Could you check a few things on this model? Use its own coordinates, in mm. A direction names the side the tool comes from. Give positions to 0.01 mm unless a question says otherwise; leave off trailing zeros. Loops run counter-clockwise (first coordinate to the right, second up) from the corner with the lowest first, then second, coordinate; pieces in that order, holes last. Notation, with made-up numbers: M 40.5,-10.5 L 70.5,-10.5 A13 ccw 70.5,-6.5 Z; hole C -37.75,20 d10. An arc over 180 degrees is marked long. Use a Markdown table: item, result. Add a question column.
1) We'd pull the mould along X, two halves only. Please class faces 1 (the conical face through (42.2, -134, -9.49)), 2 (the flat face through (97.95, -168.89, -79.07)), 3 (the flat face through (85, -148, -74)): +X half, -X half, draft (parallel to the pull), parting line (faces both ways), or undercut.
2) Suppose I cut it at A-A on x = 0. List the corners of the cut face in (y, z) for me, and give its area (3 significant figures).
3) If I drill on line 1 along Z through (x, y) = (-28, -61); line 2 along Z through (x, y) = (-81.5, -109.5); line 3 along X through (y, z) = (111, -77), over which ranges is the centre line in solid material (lowest first)? Write a range as [from, to].
4) Which directions (+Z, -Z, +X, -X, +Y, -Y) give clear straight access to the entire face, cutting with the end or side of a thin tool? Please do faces 4 (the flat face through (106, 118, -19)), 5 (the flat face through (112.732, 120.258, -59.177)), 6 (the flat face through (-155, -33, -19)), 7 (the flat face through (-161, 37.5, -58)).
5) Suppose I cut it at C-C on x = -170.5. List the corners of the cut face in (y, z) for me, and give its area (3 significant figures).
6) Will these pins go through, and if not, where does the flat tip stop? pin 1 Ø12 at (x, y) = (-144.5, 32.5) entering from +Z; pin 2 Ø5 at (x, z) = (-40, -2) entering from +Y; pin 3 Ø15 at (x, y) = (47, -147) entering from +Z.
7) Suppose I cut it at B-B on z = -49. List the corners of the cut face in (x, y) for me.
```python
from build123d import *

# Parameters (mm, degrees)
SKETCH1_R                    = 150
BOSS_EXTRUDE1_DEPTH          = 75
CHAMFER1_SIZE                = 10
BOSS_EXTRUDE2_START          = -75
BOSS_EXTRUDE2_DEPTH          = 10
CHAMFER2_SIZE                = 10
BOSS_EXTRUDE3_DEPTH          = 10
CIRPATTERN2_COUNT            = 3
CIRPATTERN2_COPY_1_DEPTH     = 10
CIRPATTERN2_COPY_2_DEPTH     = 10
CHAMFER2_OF_CIRPATTERN2_SIZE = 10
SKETCH4_R                    = 110
BOSS_EXTRUDE4_DEPTH          = 9
BOSS_EXTRUDE4_TAPER          = 45
SKETCH5_R                    = 10
BOSS_EXTRUDE5_DEPTH          = 20
BODY_MOVE_COPY1_ANGLE        = 90


with BuildPart() as part:
    # Sketch1 → Boss-Extrude1 (new body)
    with BuildSketch(Plane(origin=(0, 0, 0), x_dir=(1, 0, 0), z_dir=(0, 1, 0))):
        with Locations(Location((0, 0, 0), (0, 0, 270))):
            Circle(SKETCH1_R)
    extrude(amount=BOSS_EXTRUDE1_DEPTH)

    # Chamfer1
    chamfer1_edges = [part.edges().sort_by_distance(p)[0] for p in [
        (0, 75, -150),
    ]]
    chamfer(chamfer1_edges, length=CHAMFER1_SIZE)

    # Sketch2 → Boss-Extrude2 (add)
    with BuildSketch(Plane(origin=(0, 75, 0), x_dir=(1, 0, 0), z_dir=(0, 1, 0)).offset(BOSS_EXTRUDE2_START)):
        with BuildLine():
            Line((-195.236875483, -37.5), (-195.236875483, 37.5))
            Line((-195.236875483, 37.5), (-145.236875483, 37.5))
            ThreePointArc((-145.236875483, 37.5), (-150, 0), (-145.236875483, -37.5))
            Line((-145.236875483, -37.5), (-195.236875483, -37.5))
        make_face()
    boss_extrude2 = extrude(amount=BOSS_EXTRUDE2_DEPTH)

    # Chamfer2
    chamfer2_edges = [part.edges().sort_by_distance(p)[0] for p in [
        (-195.236875483, 5, -37.5),
        (-195.236875483, 5, 37.5),
    ]]
    chamfer(chamfer2_edges, length=CHAMFER2_SIZE)

    # Sketch3 → Boss-Extrude3 (add)
    with BuildSketch(Plane.XY.offset(37.5)):
        Polygon((-145.236875483, 10), (-145.236875483, 65), (-165.236875483, 65), (-185.236875483, 10), align=None)
    boss_extrude3 = extrude(amount=-BOSS_EXTRUDE3_DEPTH)

    # Mirror3: Boss-Extrude3 across plane
    add(boss_extrude3.mirror(Plane.XY))

    # CirPattern2: Boss-Extrude2, Boss-Extrude3 ×3 about axis
    cirpattern2_axis = Axis((0, 0, 0), (0, 1, 0))
    add([boss_extrude2.rotate(cirpattern2_axis, i * 360 / CIRPATTERN2_COUNT) for i in range(1, CIRPATTERN2_COUNT)])
    add([boss_extrude3.rotate(cirpattern2_axis, i * 360 / CIRPATTERN2_COUNT) for i in range(1, CIRPATTERN2_COUNT)])

    # CirPattern2 copy 1 sketch → CirPattern2 copy 1 (add)
    with BuildSketch(Plane(origin=(-32.475952642, 0, 18.75), x_dir=(-0.4999999999999998, 0, -0.8660254037844387), z_dir=(-0.8660254037844387, 0, 0.4999999999999998))):
        Polygon((-145.236875483, -10), (-145.236875483, -65), (-165.236875483, -65), (-185.236875483, -10), align=None)
    extrude(amount=-CIRPATTERN2_COPY_1_DEPTH)

    # CirPattern2 copy 2 sketch → CirPattern2 copy 2 (add)
    with BuildSketch(Plane(origin=(32.475952642, 0, 18.75), x_dir=(-0.5000000000000004, 0, 0.8660254037844384), z_dir=(0.8660254037844384, 0, 0.5000000000000004))):
        Polygon((-145.236875483, -10), (-145.236875483, -65), (-165.236875483, -65), (-185.236875483, -10), align=None)
    extrude(amount=-CIRPATTERN2_COPY_2_DEPTH)

    # Chamfer2 of CirPattern2
    chamfer2_of_cirpattern2_edges = [part.edges().sort_by_distance(p)[0] for p in [
        (65.142485099, 5, 187.830093924),
        (130.094390383, 5, 150.330093924),
        (130.094390383, 5, -150.330093924),
        (65.142485099, 5, -187.830093924),
    ]]
    chamfer(chamfer2_of_cirpattern2_edges, length=CHAMFER2_OF_CIRPATTERN2_SIZE)

    # Sketch4 → Boss-Extrude4 (add)
    with BuildSketch(Plane(origin=(0, 75, 0), x_dir=(1, 0, 0), z_dir=(0, 1, 0))):
        Circle(SKETCH4_R)
    extrude(amount=BOSS_EXTRUDE4_DEPTH, taper=BOSS_EXTRUDE4_TAPER)

    # Sketch5 → Boss-Extrude5 (add)
    with BuildSketch(Plane(origin=(0, 84, 0), x_dir=(1, 0, 0), z_dir=(0, 1, 0))):
        with Locations(Location((0, 0, 0), (0, 0, 270))):
            Circle(SKETCH5_R)
    extrude(amount=BOSS_EXTRUDE5_DEPTH)


with BuildPart() as part_1:
    # Body-Move/Copy1: read off the stored shape, not the designer's step
    # Body-Move/Copy1: moved
    add(part.part.rotate(Axis((0, 0, 0), (1, 0, 0)), BODY_MOVE_COPY1_ANGLE))


with BuildPart() as part_2:
    # Body-Move/Copy2: moved
    add(part_1.part.moved(Location((5e-08, 0, -83.99999995))))


solid = part_2.part
```
Answer block:
| question | item | result |
|---|---|---|
| 1 | face 1 | parting line |
| 1 | face 2 | +X half |
| 1 | face 3 | undercut |
| 2 | outline | M -150,-84 L 150,-84 L 150,-19 L 140,-9 L 110,-9 L 101,0 L 10,0 L 10,20 L -10,20 L -10,0 L -101,0 L -110,-9 L -140,-9 L -150,-19 Z |
| 2 | area | 24,700 mm^2 |
| 3 | line 1 | z = [-84, 0] |
| 3 | line 2 | z = [-84, -9] |
| 3 | line 3 | x = [-100.89, 107.39] |
| 4 | face 4 | +Z, +X, +Y |
| 4 | face 5 | +Z, -Z, +X |
| 4 | face 6 | +Z, -X, -Y |
| 4 | face 7 | +Z, -Z, -X, +Y |
| 5 | outline | M -37.5,-84 L 37.5,-84 L 37.5,-33.47 L 27.5,-33.47 L 27.5,-74 L -27.5,-74 L -27.5,-33.47 L -37.5,-33.47 Z |
| 5 | area | 1,560 mm^2 |
| 6 | pin 1 | stops at z = -11.11 |
| 6 | pin 2 | stops at y = 97.81 |
| 6 | pin 3 | stops at z = -15.83 |
| 7 | outline | M -176.15,-37.5 L -145.24,-37.5 A150 ccw 40.14,-144.53 L 55.6,-171.3 L 64.26,-166.3 L 49.91,-141.45 A150 ccw 97.54,-113.95 L 111.89,-138.8 L 120.55,-133.8 L 105.09,-107.03 A150 ccw 105.09,107.03 L 120.55,133.8 L 111.89,138.8 L 97.54,113.95 A150 ccw 49.91,141.45 L 64.26,166.3 L 55.6,171.3 L 40.14,144.53 A150 ccw -145.24,37.5 L -176.15,37.5 L -176.15,27.5 L -147.46,27.5 A150 ccw -147.46,-27.5 L -176.15,-27.5 Z |
